Design review of the part shown in the three views and the two pictorial views. Dimensions are in mm from the part's minimum x, y and z. A direction names the side the tool comes from. Give positions to 0.01 mm unless a question says otherwise; leave off trailing zeros. Order: outer loops, then holes, each group sorted by start corner. A loop starts at its lowest first (then second) coordinate and runs counter-clockwise, first axis right, second up. Notation, with made-up numbers: (82, 40.5) - (140, 40.5) arc R35 ccw to (140, 78.5) - close; hole circle Ø9 at (-15, 26.5). An arc over 180 degrees is marked (long way). Put each result on its own line as item: value. Start each with the question number.
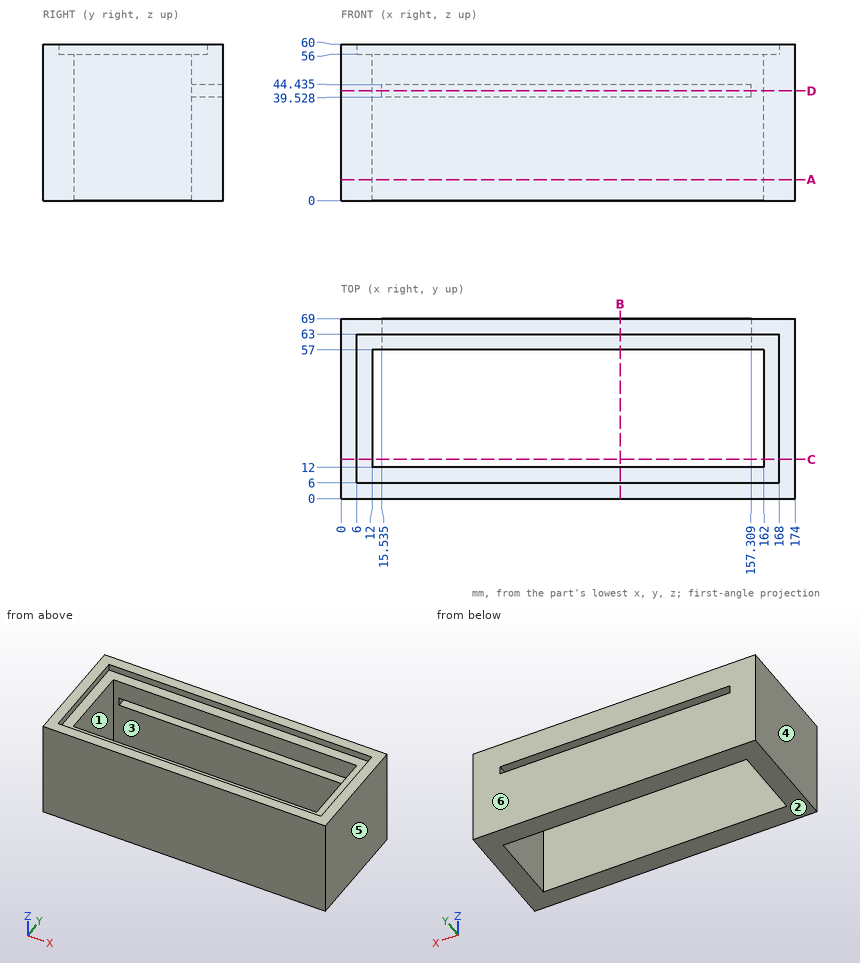
1. Add section C-C, the plane y = 15. Give the boundary of the cut face in (x, z), then the cut area to 3 significant figures.
2. Wall thickness on line 1 (X direction, y = 25.5, z = 12.5); line 2 (Y direction, x = 17.5, z = 8); line 3 (Z direction, x = 48, y = 6.5): over which ranges is each line inside the solid? List them lowest first. Write a range as from..to.
3. Add section A-A, the plane z = 8. Give the boundary of the cut face in (x, y).
4. Tool access review of the marked faces 1 and 2: name each direction out of +Z, -Z, +X, -X, +Y, -Y from which nothing blocks a thin tool from reaching the whole face with its end or side.
5. Add section D-D, the plane z = 42. Give the boundary of the cut face in (x, y) (1 decimal).
6. Add section B-B, the plane x = 107. Give the boundary of the cut face in (y, z) (1 decimal), then the cut area to 3 significant figures.
7. The part is to be moulded in two halves that separate along X. For the marked faces 3, 4, 5 and 6, say which applies: released by +X, released by -X, zero draft, split by the parting line, or undercut.
Found:
1. outline: (0, 0) - (12, 0) - (12, 56) - (6, 56) - (6, 60) - (0, 60) - close; (162, 0) - (174, 0) - (174, 60) - (168, 60) - (168, 56) - (162, 56) - close
1. area: 1,390 mm^2
2. line 1: x = 0..12, 162..174
2. line 2: y = 0..12, 57..69
2. line 3: z = 0..56
3. outline: (0, 0) - (174, 0) - (174, 69) - (0, 69) - close; hole (12, 12) - (162, 12) - (162, 57) - (12, 57) - close
4. face 1: +Z, -Z
4. face 2: -Z, +X, -X, +Y, -Y
5. outline: (0, 0) - (174, 0) - (174, 69) - (157.3, 69) - (157.3, 57) - (162, 57) - (162, 12) - (12, 12) - (12, 57) - (15.5, 57) - (15.5, 69) - (0, 69) - close
6. outline: (0, 0) - (12, 0) - (12, 56) - (6, 56) - (6, 60) - (0, 60) - close; (57, 0) - (69, 0) - (69, 39.5) - (57, 39.5) - close; (57, 44.4) - (69, 44.4) - (69, 60) - (63, 60) - (63, 56) - (57, 56) - close
6. area: 1,330 mm^2
7. face 3: undercut
7. face 4: released by -X
7. face 5: released by +X
7. face 6: zero draft
